Autodesk Inventor part; units mm, degrees
ref_plane "YZ Plane" through (0, 0, 0) normal (1, 0, 0) x (0, 1, 0)
ref_plane "XZ Plane" through (0, 0, 0) normal (0, 1, 0) x (-1, 0, 0)
ref_plane "XY Plane" through (0, 0, 0) normal (0, 0, 1) x (1, 0, 0)
sketch "スケッチ1" plane through (0, 0, 0) normal (1, 0, 0) x (0, 1, 0)
  line L0 (-10.5, -10) -> (10.5, -10)
  line L1 (10.5, -10) -> (10.5, 10)
  line L2 (10.5, 10) -> (-10.5, 10)
  line L3 (-10.5, 10) -> (-10.5, -10)
  line L4 (-10.5, -10) -> (10.5, 10) construction
  line L5 (10.5, -10) -> (-10.5, 10) construction
  point P0 (0, 0)
  dimension "d0" = 21
  dimension "d1" = 20
extrude "プレート1" add sketch "スケッチ1" along normal blind 2
sketch "スケッチ3" plane through (2.0304, -10.8473, -10) normal (-0.9848078, -0.1736482, 0) x (0.1736482, -0.9848078, 0)
  line L0 (0, 20) -> (0, 0)
  line L1 (0, 0) -> (24.65, 0)
  line L2 (24.65, 0) -> (24.65, 20)
  line L3 (24.65, 20) -> (0, 20)
edge flange "フランジ2" height 25 angle 10 thickness 2 bend radius 2 thickness toward (-0.9848078, -0.1736482, 0) relief tear relief width 2 relief depth 1 edges at (2, -10.5, 0) wall of the first edge with corners at (2.0304, -10.8473, 10) (2.0304, -10.8473, -10) (6.3108, -35.1229, -10) (6.3108, -35.1229, 10)
bend "曲げ2"
corner "コーナー2"
sketch "スケッチ5" plane through (2, 0, 0) normal (1, 0, 0) x (0, 0, -1)
  line L0 (7, -7) -> (-7, -7)
  line L1 (-7, -7) -> (-7, 7)
  line L2 (-7, 7) -> (7, 7)
  line L3 (7, 7) -> (7, -7)
  line L4 (7, -7) -> (-7, 7) construction
  line L5 (-7, -7) -> (7, 7) construction
  point P0 (0, 0)
  dimension "d27" = 14
  dimension "d28" = 14
extrude "押し出し2" cut sketch "スケッチ5" against normal blind 10
sketch "スケッチ6" plane through (6.3108, -35.1229, 10) normal (0.9848078, 0.1736482, 0) x (0, 0, -1)
  line L0 (17, 5.325) -> (3, 5.325)
  line L1 (3, 5.325) -> (3, 19.325)
  line L2 (3, 19.325) -> (17, 19.325)
  line L3 (17, 19.325) -> (17, 5.325)
  line L4 (17, 5.325) -> (3, 19.325) construction
  line L5 (3, 5.325) -> (17, 19.325) construction
  line L6 (20, 0) -> (20, 24.65)
  line L7 (17, 28.4442) -> (3, 28.4442)
  point P0 (10, 35.6851)
  point P1 (10, 12.325)
  point P2 (10, 12.325)
  point P3 (20, 12.325)
  point P4 (10, 12.325)
  point P5 (10, 28.4442)
  dimension "d31" = 14
  dimension "d32" = 14
extrude "押し出し3" cut sketch "スケッチ6" against normal blind 10
sketch "スケッチ7" plane through (7.5964, -36.6549, 10) normal (-0.3420201, -0.9396926, 0) x (-0.9396926, 0.3420201, 0)
  line L0 (0, -20) -> (0, 0)
  line L1 (0, 0) -> (-8.8453, 0)
  line L2 (-8.8453, 0) -> (-8.8453, -20)
  line L3 (-8.8453, -20) -> (0, -20)
edge flange "フランジ3" height 10 angle -60 thickness 2 bend radius 2 thickness toward (-0.3420201, -0.9396926, 0) relief tear relief width 2 relief depth 1 edges at (4.3412, -35.4701, 0) wall of the first edge with corners at (7.5964, -36.6549, -10) (7.5964, -36.6549, 10) (15.9083, -39.6802, 10) (15.9083, -39.6802, -10)
bend "曲げ3"
corner "コーナー3"
sketch "スケッチ8" plane through (15.9083, -39.6802, 10) normal (0.3420201, 0.9396926, 0) x (0.9396926, -0.3420201, 0)
  line L0 (-5.9226, 4) -> (-5.9226, 16)
  arc A0 (-2.9226, 16) -> (-5.9226, 16) centre (-4.4226, 16) ccw
  line L1 (-2.9226, 16) -> (-2.9226, 4)
  arc A1 (-5.9226, 4) -> (-2.9226, 4) centre (-4.4226, 4) ccw
  line L2 (-8.8453, 20) -> (0, 20)
  line L3 (0, 0) -> (-8.8453, 0)
  point P0 (-28.5203, 10)
  point P1 (-4.4226, 20)
  dimension "d45" = 4
  dimension "d46" = 4
  dimension "d47" = 1.5
extrude "押し出し4" cut sketch "スケッチ8" against normal blind 10
sketch "スケッチ25" plane through (-2, 12.5, -10) normal (0, 1, 0) x (-1, 0, 0)
  line L0 (0, 20) -> (0, 0)
  line L1 (0, 0) -> (8, 0)
  line L2 (8, 0) -> (8, 20)
  line L3 (8, 20) -> (0, 20)
edge flange "フランジ12" height 10 angle 90 thickness 2 bend radius 2 thickness toward (0, 1, 0) relief tear relief width 2 relief depth 1 edges at (0, 10.5, 0) wall of the first edge with corners at (-2, 12.5, 10) (-2, 12.5, -10) (-10, 12.5, -10) (-10, 12.5, 10)
bend "曲げ21"
corner "コーナー12"
sketch "スケッチ26" plane through (-11.9696, 10.8473, -10) normal (-0.9848078, 0.1736482, 0) x (-0.1736482, -0.9848078, 0)
  line L0 (0, 20) -> (0, 0)
  line L1 (0, 0) -> (37.0268, 0)
  line L2 (37.0268, 0) -> (37.0268, 20)
  line L3 (37.0268, 20) -> (0, 20)
edge flange "フランジ13" height 38.705 angle 80 thickness 2 bend radius 2 thickness toward (-0.9848078, 0.1736482, 0) relief tear relief width 2 relief depth 1 edges at (-10, 12.5, 0) wall of the first edge with corners at (-11.9696, 10.8473, 10) (-11.9696, 10.8473, -10) (-18.3993, -25.617, -10) (-18.3993, -25.617, 10)
bend "曲げ22"
corner "コーナー13"
sketch "スケッチ27" plane through (-17.1137, -27.8437, -10) normal (-0.3420201, -0.9396926, 0) x (0.9396926, -0.3420201, 0)
  line L0 (0, 20) -> (0, 0)
  line L1 (0, 0) -> (8.3218, 0)
  line L2 (8.3218, 0) -> (8.3218, 20)
  line L3 (8.3218, 20) -> (0, 20)
edge flange "フランジ14" height 10 angle 80 thickness 2 bend radius 2 thickness toward (-0.3420201, -0.9396926, 0) relief tear relief width 2 relief depth 1 edges at (-18.3993, -25.617, 0) wall of the first edge with corners at (-17.1137, -27.8437, 10) (-17.1137, -27.8437, -10) (-9.2937, -30.6899, -10) (-9.2937, -30.6899, 10)
bend "曲げ23"
corner "コーナー14"
sketch "スケッチ28" plane through (-9.2937, -30.6899, 10) normal (0.3420201, 0.9396926, 0) x (0.9396926, -0.3420201, 0)
  line L0 (-5.6609, 4) -> (-5.6609, 16)
  arc A0 (-2.6609, 16) -> (-5.6609, 16) centre (-4.1609, 16) ccw
  line L1 (-2.6609, 16) -> (-2.6609, 4)
  line L2 (-2.2781, 3) -> (-2.2781, 17)
  arc A1 (-5.6609, 4) -> (-2.6609, 4) centre (-4.1609, 4) ccw
  line L3 (0, 0) -> (-8.3218, 0)
  line L4 (0, 20) -> (-8.3218, 20)
  point P0 (-1.7633, 10)
  point P1 (-4.1609, 20)
  dimension "d224" = 4
  dimension "d225" = 4
  dimension "d226" = 1.5
extrude "押し出し6" cut sketch "スケッチ28" against normal blind 10
equation "\"d2\" = Thickness"
equation "\"d13\" = BendReliefWidth"
equation "\"d14\" = BendReliefDepth"
equation "\"d15\" = MinimumRemnant"
equation "\"d16\" = TransitionRadius"
equation "\"d19\" = BendRadius"
equation "\"d20\" = CornerReliefSize"
equation "\"d21\" = GapSize"
equation "\"d22\" = JacobiRadiusSize"
equation "\"d35\" = BendReliefWidth"
equation "\"d36\" = BendReliefDepth"
equation "\"d37\" = MinimumRemnant"
equation "\"d38\" = TransitionRadius"
equation "\"d41\" = BendRadius"
equation "\"d42\" = CornerReliefSize"
equation "\"d43\" = GapSize"
equation "\"d44\" = JacobiRadiusSize"
equation "\"d194\" = BendReliefWidth"
equation "\"d195\" = BendReliefDepth"
equation "\"d196\" = MinimumRemnant"
equation "\"d197\" = TransitionRadius"
equation "\"d200\" = BendRadius"
equation "\"d201\" = CornerReliefSize"
equation "\"d202\" = GapSize"
equation "\"d203\" = JacobiRadiusSize"
equation "\"d204\" = BendReliefWidth"
equation "\"d205\" = BendReliefDepth"
equation "\"d206\" = MinimumRemnant"
equation "\"d207\" = TransitionRadius"
equation "\"d210\" = BendRadius"
equation "\"d211\" = CornerReliefSize"
equation "\"d212\" = GapSize"
equation "\"d213\" = JacobiRadiusSize"
equation "\"d214\" = BendReliefWidth"
equation "\"d215\" = BendReliefDepth"
equation "\"d216\" = MinimumRemnant"
equation "\"d217\" = TransitionRadius"
equation "\"d220\" = BendRadius"
equation "\"d221\" = CornerReliefSize"
equation "\"d222\" = GapSize"
equation "\"d223\" = JacobiRadiusSize"
equation "\"BendRadius\" = Thickness"
equation "\"BendReliefWidth\" = Thickness"
equation "\"BendReliefDepth\" = 0.5 * Thickness"
equation "\"CornerReliefSize\" = 4 * Thickness"
equation "\"MinimumRemnant\" = 2 * Thickness"
equation "\"TransitionRadius\" = BendRadius"
equation "\"JacobiRadiusSize\" = BendRadius"
equation "\"GapSize\" = Thickness"
properties part number "ThumbPlate" material "アルミニウム 6061"
Check sheet for the modelled part. Datum: model origin and axes. Units: mm. A direction names the side the tool comes from. Coordinates: 2 decimals unless noted, no trailing zeros. Loops run counter-clockwise (first coordinate to the right, second up) from the corner with the lowest first, then second, coordinate; pieces in that order, holes last. Notation, with made-up numbers: (38, -10) -> (46, -10) arc R24 cw to (46, 28) -> close; hole circle Ø2 at (-25, -16). An arc over 180 degrees is marked (long way). Write item = value, one per line. Start each with the question number.
1. Depth check by flat-ended pin: P1, Ø10, axis at y = -34.5, z = -6, coming from the -X side; P2, Ø6, axis at x = -1, y = -26.5, coming from the -Z side; P3, Ø2, axis at y = -34.5, z = 2.5, coming from the +X side; P4, Ø6, axis at x = 9.5, z = 5.5, coming from the +Y side. Enter the tip coordinate at first touch or a pass-through.
2. Material ranges on line 1 (X direction, y = -11, z = 2.5); line 2 (Y direction, x = -8, z = 1); line 3 (X direction, y = -13.5, z = -2.5), recorded low to high.
3. Section check C-C on z = -8.5. Record the cut outline in (x, y), then the cut area to 3 significant figures.
4. Section check D-D on x = -6.5. Record the cut outline in (y, z).
5. Tool access check on faces 1 (the cylindrical face through (-18.152, -26.981, -0.14)), 2 (the flat face through (1.984, -16.263, 0.098)), 3 (the flat face through (-9.631, -31.616, -0.14)), 4 (the flat face through (4.42, -30.05, -0.1)). Record the directions out of +Z, -Z, +X, -X, +Y, -Y that give a thin tool (end or side, any length) a straight path to the whole face; none if there is none.
6. Draft check along X on faces 5 (the flat face through (1, 0, 7)), 6 (the flat face through (0, -7.15, 0.14)), 7 (the cylindrical face through (0.797, 13.359, -0.14)). Enter one of: released by +X, released by -X, zero draft, split by the parting line, or undercut.
7. Section check A-A on y = -2. Record the cut outline in (x, z).
8. Section check B-B on y = -9.5. Record the cut outline in (x, z).
Responses:
q1.P1 = -18.3
q1.P2 = through
q1.P3 = 6.42
q1.P4 = -35.69
q2.line_1 = -17.85 to -15.82, 0.03 to 2.06
q2.line_2 = 12.5 to 14.5
q2.line_3 = -18.29 to -16.26, 0.47 to 2.5
q3.outline = (-20.37, -25.27) arc R4 ccw to (-17.8, -29.72) -> (-9.98, -32.57) -> (-9.29, -30.69) -> (-17.11, -27.84) arc R2 cw to (-18.4, -25.62) -> (-11.97, 10.85) arc R2 cw to (-10, 12.5) -> (-2, 12.5) arc R2 cw to (0, 10.5) -> (0, -10.5) arc R4 ccw to (0.06, -11.19) -> (4.34, -35.47) arc R4 ccw to (6.91, -38.53) -> (15.22, -41.56) -> (15.91, -39.68) -> (7.6, -36.65) arc R2 cw to (6.31, -35.12) -> (2.03, -10.85) arc R2 cw to (2, -10.5) -> (2, 10.5) arc R4 ccw to (-2, 14.5) -> (-10, 14.5) arc R4 ccw to (-13.94, 11.19) -> close
q3.area = 249 mm2
q4.outline = (12.5, -10) -> (14.5, -10) -> (14.5, 10) -> (12.5, 10) -> close
q5.face_1 = +Z, -Z
q5.face_2 = +X, -Y
q5.face_3 = +Z, -Z, -Y
q5.face_4 = +Y
q6.face_5 = zero draft
q6.face_6 = undercut
q6.face_7 = released by +X
q7.outline = (-16.27, -10) -> (-14.23, -10) -> (-14.23, 10) -> (-16.27, 10) -> close; (0, -10) -> (2, -10) -> (2, -7) -> (0, -7) -> close; (0, 7) -> (2, 7) -> (2, 10) -> (0, 10) -> close
q8.outline = (-17.59, -10) -> (-15.56, -10) -> (-15.56, 10) -> (-17.59, 10) -> close; (0, -10) -> (2, -10) -> (2, 10) -> (0, 10) -> close
